Geometry: final body of the model. Coordinates: model frame, mm. A direction names the side the tool comes from. Coordinates: 2 decimals unless noted, no trailing zeros. Order: outer loops, then holes, each group sorted by start corner. A loop starts at its lowest first (then second) coordinate and runs counter-clockwise, first axis right, second up. Notation, with made-up numbers: (34.5, 14) - (54.5, 14) arc R32 cw to (54.5, 50) - close; hole circle Ø11 at (52, -27). An arc over 180 degrees is marked (long way). Use a Markdown table: item, result. Add a question column.
```python
from build123d import *

# Parameters (mm, degrees)
SKETCH3_W               = 1.121172813
SKETCH3_H               = 3
BOSS_EXTRUDE1_DEPTH     = 3
SKETCH4_W               = 4
SKETCH4_H               = 1
BOSS_EXTRUDE2_DEPTH     = 3
FILLET3_R               = 1
CUT_EXTRUDE4_DEPTH      = 6.127147937
CUT_EXTRUDE4_DEPTH_BACK = 6.127147937
CUT_EXTRUDE5_DEPTH      = 6.830951895
BOSS_EXTRUDE4_REACH     = 11.163
SKETCH26_W              = 3
SKETCH26_H              = 1
FILLET6_R               = 1
SKETCH27_R              = 0.25
CUT_EXTRUDE6_DEPTH      = 10.614711327
CUT_EXTRUDE7_DEPTH      = 8.660792968
CUT_EXTRUDE7_DEPTH_BACK = 8.660792968
SKETCH28_R              = 0.5
FILLET7_R               = 0.5


with BuildPart() as part:
    # Sketch3 → Boss-Extrude1 (new body)
    with BuildSketch(Plane(origin=(0, 0, 0), x_dir=(1, 0, 0), z_dir=(0, 1, 0))):
        with Locations((0.560586407, -1.5)):
            Rectangle(SKETCH3_W, SKETCH3_H)
    extrude(amount=BOSS_EXTRUDE1_DEPTH)

    # Sketch4 → Boss-Extrude2 (add)
    with BuildSketch(Plane.XY):
        with Locations((2, 0.5)):
            Rectangle(SKETCH4_W, SKETCH4_H)
    extrude(amount=BOSS_EXTRUDE2_DEPTH)

    # Fillet3
    fillet3_edges = [part.edges().sort_by_distance(p)[0] for p in [
        (0.560586407, 3, 0),
        (0.560586407, 3, 3),
    ]]
    fillet(fillet3_edges, radius=FILLET3_R)

    # Sketch5 → Cut-Extrude4 (cut, two sides: drawn at the far end of the back side and taken through both)
    with BuildSketch(Plane(origin=(1.121172813, 0, 0), x_dir=(0, 0, -1), z_dir=(1, 0, 0)).offset(-CUT_EXTRUDE4_DEPTH_BACK)):
        with BuildLine():
            ThreePointArc((-1.75, 2), (-2, 2.25), (-2.25, 2))
            Line((-2.25, 2), (-1.75, 2))
        make_face()
        with BuildLine():
            Line((-1.75, 2), (-2.25, 2))
            ThreePointArc((-2.25, 2), (-2, 1.75), (-1.75, 2))
        make_face()
        with BuildLine():
            ThreePointArc((-0.75, 2), (-1, 2.25), (-1.25, 2))
            Line((-1.25, 2), (-0.75, 2))
        make_face()
        with BuildLine():
            Line((-0.75, 2), (-1.25, 2))
            ThreePointArc((-1.25, 2), (-1, 1.75), (-0.75, 2))
        make_face()
    extrude(amount=CUT_EXTRUDE4_DEPTH + CUT_EXTRUDE4_DEPTH_BACK, mode=Mode.SUBTRACT)

    # Sketch12 → Cut-Extrude5 (cut, through all)
    with BuildSketch(Plane.XZ):
        Polygon((4, 0), (3.000287903, 3), (4, 3), align=None)
    extrude(amount=-CUT_EXTRUDE5_DEPTH, mode=Mode.SUBTRACT)

    # Sweep1: read off the stored shape, not the designer's step
    # Sweep1: loft between two sections, ruled curve by curve
    sweep1_from = [
        Edge.make_line((5.182299836, -1.182011934, 3), (5.182299836, -2.182011934, 3)),
        Edge.make_line((3.000287903, 1, 3), (5.182299836, -1.182011934, 3)),
        Edge.make_line((5.182299836, -2.182011934, 3), (3.000287903, 0, 3)),
        Edge.make_line((3.000287903, 0, 3), (3.000287903, 1, 3)),
    ]
    sweep1_to = [
        Edge.make_line((6.182011934, -1.182011934, 0), (6.182011934, -2.182011934, 0)),
        Edge.make_line((4, 1, 0), (6.182011934, -1.182011934, 0)),
        Edge.make_line((6.182011934, -2.182011934, 0), (4, 0, 0)),
        Edge.make_line((4, 0, 0), (4, 1, 0)),
    ]
    sweep1 = Solid(Shell([*[Face.make_surface_from_curves(sweep1_from[k], sweep1_to[k]) for k in range(4)], Face(Wire(sweep1_from)), Face(Wire(sweep1_to))]))
    add(sweep1)

    # Sketch26 → Boss-Extrude4 (add, up to next)
    with BuildSketch(Plane(origin=(8.121172813, 0, 0), x_dir=(0, 0, -1), z_dir=(1, 0, 0)), mode=Mode.PRIVATE) as boss_extrude4_sk1:
        with Locations((-1.5, -1.682011934)):
            Rectangle(SKETCH26_W, SKETCH26_H)
    boss_extrude4_tool1 = extrude(boss_extrude4_sk1.sketch, amount=-BOSS_EXTRUDE4_REACH, mode=Mode.PRIVATE) - part.part
    add(boss_extrude4_tool1.solids().sort_by_distance((8.121173, -1.682012, 1.5))[0])

    # Fillet6
    fillet6_edges = [part.edges().sort_by_distance(p)[0] for p in [
        (8.121172813, -1.682011934, 0),
        (8.121172813, -1.682011934, 3),
    ]]
    fillet(fillet6_edges, radius=FILLET6_R)

    # Sketch27 → Cut-Extrude6 (cut, through all)
    with BuildSketch(Plane(origin=(0, -1.182011934, 0), x_dir=(1, 0, 0), z_dir=(0, 1, 0))):
        with Locations(Location((7.121172813, -2.25, 0), (0, 0, 270))):
            Circle(SKETCH27_R)
        with Locations(Location((7.121172813, -0.75, 0), (0, 0, 90))):
            Circle(SKETCH27_R)
    extrude(amount=-CUT_EXTRUDE6_DEPTH, mode=Mode.SUBTRACT)

    # Sketch28 → Cut-Extrude7 (cut, two sides: drawn at the far end of the back side and taken through both)
    with BuildSketch(Plane(origin=(2.368492821, 2.368492821, 0.789270309), x_dir=(0.16217717426622844, 0.16217717426622855, -0.973343273616273), z_dir=(0.6882576291963799, 0.6882576291963798, 0.2293531593546452)).offset(-CUT_EXTRUDE7_DEPTH_BACK)):
        with Locations(Location((-0.730194281, -3.310784177, 0), (0, 0, 90))):
            Circle(SKETCH28_R)
    extrude(amount=CUT_EXTRUDE7_DEPTH + CUT_EXTRUDE7_DEPTH_BACK, mode=Mode.SUBTRACT)

    # Fillet7
    fillet7_edges = [part.edges().sort_by_distance(p)[0] for p in [
        (1.121172813, 1, 1.5),
    ]]
    fillet(fillet7_edges, radius=FILLET7_R)


solid = part.part
```
1) Section query B-B (x = 2.5). Return the cut outline in (y, z).
2) Section query A-A (x = 0.5). Return the cut outline in (y, z), and give its area (3 significant figures).
3) First-contact query: pin 1 (1.5 mm diameter, centred on x = 7, z = 2.5, fed in from +Y); pin 2 (0.9 mm diameter, centred on x = 2, z = 2, fed in from -Y); pin 3 (0.8 mm diameter, centred on y = 2, z = 1, fed in from +X). Flat tips, straight axial feed; report the tip coordinate or a pass-through.
4) Line query: line 1 (Y direction, x = 0.4, z = 1); line 2 (Y direction, x = 6.75, z = 0.4); line 3 (Y direction, x = 3, z = 1.3). Output: solid intervals per line, ascending. Write a range as from..to.
5) Draft query along Y for faces 4 (the flat face through (3.6, -0.3, 3)), 5 (the cylindrical face through (4.26, -0.096, 0.988)), 6 (the flat face through (6.7, -2.182, 1.5)). Return one class per face: released by +Y, released by -Y, zero draft, split by the parting line, or undercut.
6) Section query C-C (y = -1.45). Give the number of separate pieces and of enclosed holes in the cut face, and give its area (3 significant figures).
7) Access query for faces 1 (the flat face through (8.121, -1.7, 1.5)), 2 (the flat face through (6.7, -1.182, 1.5)), 3 (the flat face through (1.121, 2.2, 1.5)). Directions: +Z, -Z, +X, -X, +Y, -Y. A direction counts if a zero-diameter tool reaches every point of the face in a straight line with its end or side. Return the directions, or none.
From the geometry:
| question | item | result |
|---|---|---|
| 1 | outline | (0, 0) - (1, 0) - (1, 3) - (0, 3) - close |
| 2 | outline | (0, 0) - (2, 0) arc R1 ccw to (3, 1) - (3, 2) arc R1 ccw to (2, 3) - (0, 3) - close; hole circle Ø0.5 at (2, 1); hole circle Ø0.5 at (2, 2) |
| 2 | area | 8.18 mm^2 |
| 3 | pin 1 | stops at y = -1.18 |
| 3 | pin 2 | stops at y = 0 |
| 3 | pin 3 | stops at x = 1.12 |
| 4 | line 1 | y = 0..1.75, 2.25..3 |
| 4 | line 2 | y = -2.18..-1.18 |
| 4 | line 3 | y = 0..1 |
| 5 | face 4 | zero draft |
| 5 | face 5 | undercut |
| 5 | face 6 | released by -Y |
| 6 | separate pieces | 1 |
| 6 | enclosed holes | 2 |
| 6 | area | 8.69 mm^2 |
| 7 | face 1 | +Z, -Z, +X, +Y, -Y |
| 7 | face 2 | +Z, +X, +Y |
| 7 | face 3 | +Z, -Z, +X, +Y |
